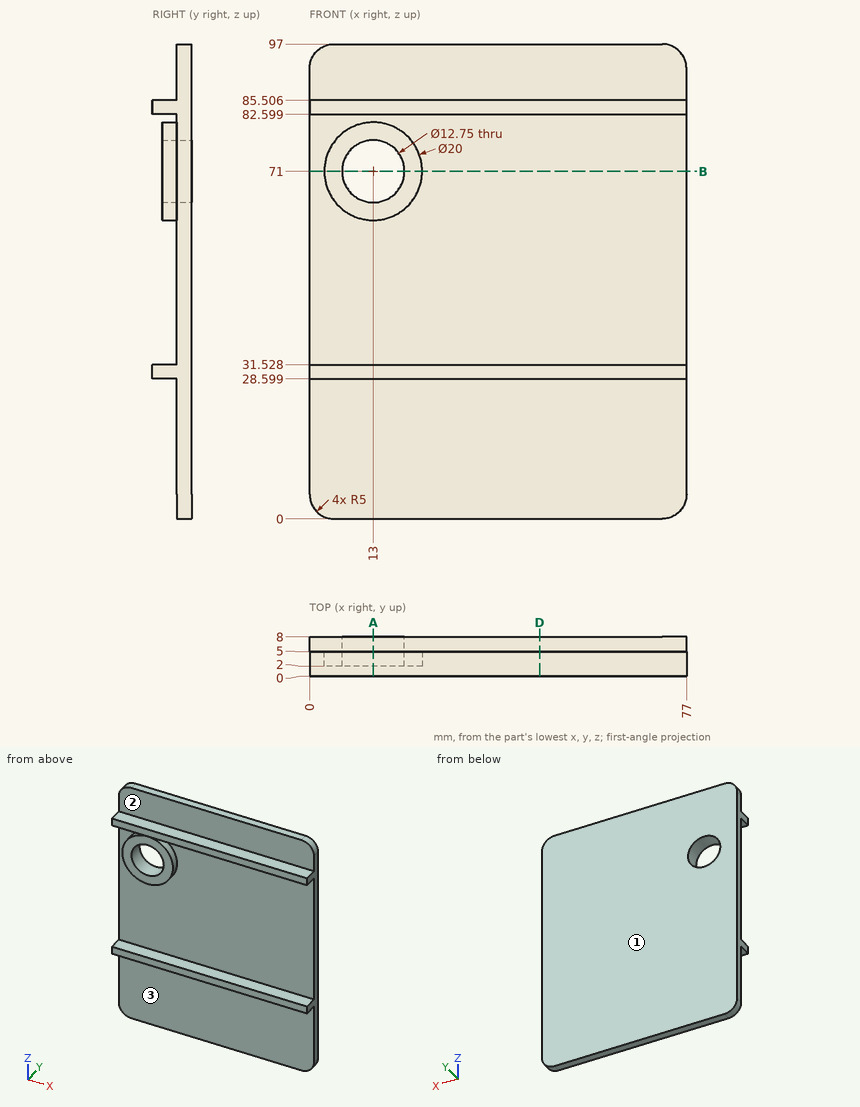
Can you work these out from the drawing? Everything is in mm from the part's minimum corner. A direction names the side the tool comes from. Coordinates: 2 decimals unless noted, no trailing zeros. Loops run counter-clockwise (first coordinate to the right, second up) from the corner with the lowest first, then second, coordinate; pieces in that order, holes last. Notation, with made-up numbers: M 28,-37 L 84,-37 A7 cw 84,-33 Z; hole C 62.25,11 d6. An arc over 180 degrees is marked long. Put each result on its own line as item: value. Start each with the question number.
(1) Suppose I cut it at D-D on x = 47. Please give me the cut outline in (y, z), then the cut area to 3 significant figures.
(2) Suppose I cut it at A-A on x = 13. Please give me the cut outline in (y, z) (1 decimal), then the cut area to 3 significant figures.
(3) For the marked faces 1, 2 and 3, which set-ups out of +Z, -Z, +X, -X, +Y, -Y let a thin tool reach every point of the face, with its end or its side?
(4) Will these pins go through, and if not, where does the flat tip stop? P1, Ø2.5, axis at x = 49.5, y = 2, coming from the -Z side; P2, Ø6, axis at x = 66, z = 77, coming from the -Y side; P3, Ø20.5, axis at x = 13, z = 71, coming from the -Y side; P4, Ø8, axis at x = 12.5, z = 76, coming from the +Y side.
(5) Suppose I cut it at B-B on z = 71. Please give me the cut outline in (x, y) (1 decimal).
(6) I need wall thicknesses on line 1 (Z direction, x = 13, y = 3.45) (1 decimal); line 2 (Z direction, x = 41, y = 2.25); line 3 (Z direction, x = 13, y = 5.85) (1 decimal). Which ranges of each line are inside material? Lowest first, please. Write a range as from..to.
Solutions:
1. outline: M 0,28.6 L 5,28.6 L 5,0 L 8,0 L 8,97 L 5,97 L 5,85.51 L 0,85.51 L 0,82.6 L 5,82.6 L 5,31.53 L 0,31.53 Z
1. area: 320 mm2
2. outline: M 0,28.6 L 5,28.6 L 5,0 L 8,0 L 8,64.6 L 2,64.6 L 2,61 L 5,61 L 5,31.5 L 0,31.5 Z; M 0,82.6 L 5,82.6 L 5,81 L 2,81 L 2,77.4 L 8,77.4 L 8,97 L 5,97 L 5,85.5 L 0,85.5 Z
2. area: 304 mm2
3. face 1: +Z, -Z, +X, -X, +Y
3. face 2: +Z, +X, -X, -Y
3. face 3: -Z, +X, -X, -Y
4. P1: stops at z = 28.6
4. P2: stops at y = 5
4. P3: stops at y = 2
4. P4: stops at y = 8
5. outline: M 0,5 L 3,5 L 3,2 L 6.6,2 L 6.6,8 L 0,8 Z; M 19.4,2 L 23,2 L 23,5 L 77,5 L 77,8 L 19.4,8 Z
6. line 1: z = 28.6..31.5, 61..64.6, 77.4..81, 82.6..85.5
6. line 2: z = 28.6..31.53, 82.6..85.51
6. line 3: z = 0..64.6, 77.4..97
